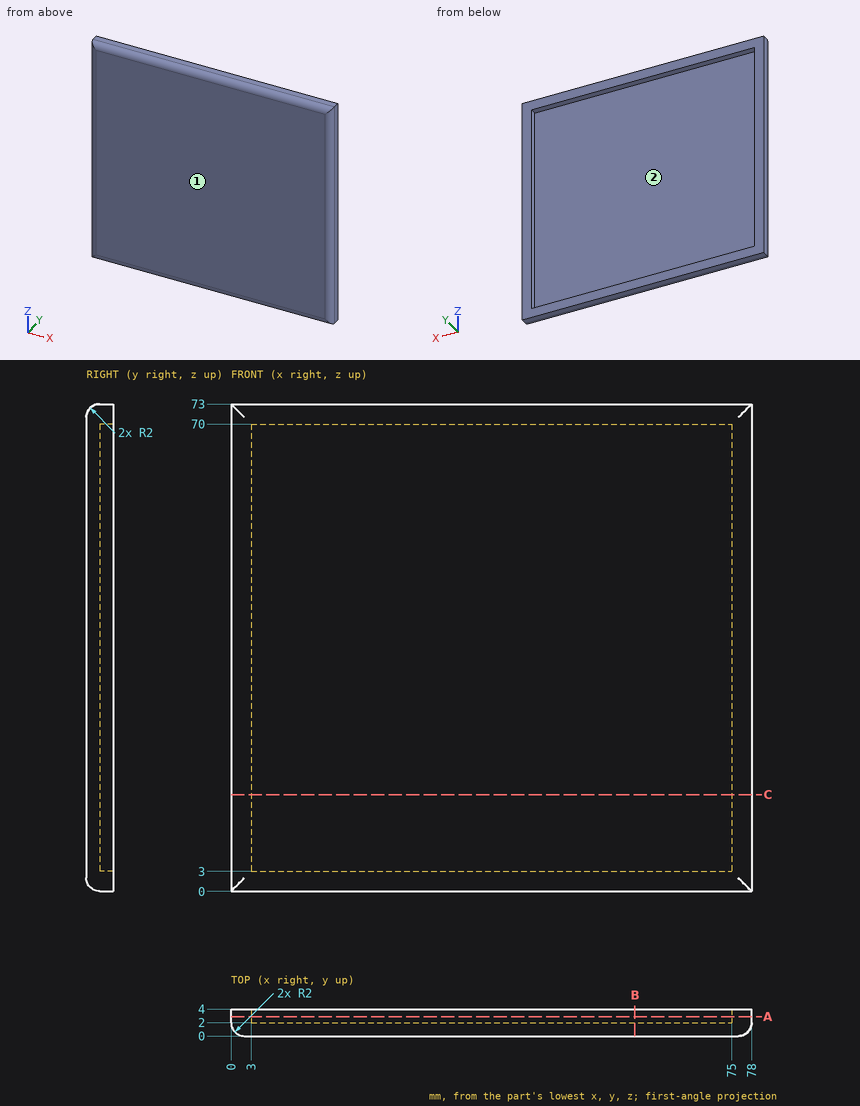
Study the drawing (mm; zero at the part's minimum x, y, z) and answer. Give positions to 0.01 mm unless a question says otherwise; leave off trailing zeros. Loops run counter-clockwise (first coordinate to the right, second up) from the corner with the lowest first, then second, coordinate; pieces in that order, holes last. Notation, with made-up numbers: M -23,3.5 L -8,3.5 A26 cw -8,39.5 Z; hole C 22,-31.75 d6. An arc over 180 degrees is marked long. Answer as CSV lines item,"result".
Item 1: Straight lines are drawn through the part: line 1 along Z through (x, y) = (23.5, 3.55); line 2 along X through (y, z) = (2.65, 45.5); line 3 along Y through (x, z) = (24.5, 5). For each, find the intervals that lie inside material, in ascending order. Write a range as [from, to].
Values follow:
line 1,"z = [0, 3], [70, 73]"
line 2,"x = [0, 3], [75, 78]"
line 3,"y = [0, 2]"
Item 2: The part is cut by section A-A (y = 2.9). Give the vertices of the cut face in (x, z).
Values follow:
outline,"M 0,0 L 78,0 L 78,73 L 0,73 Z; hole M 3,3 L 75,3 L 75,70 L 3,70 Z"
Item 3: The part is cut by section B-B (x = 60.5). Give the vertices of the cut face in (y, z), and give its area (3 significant figures).
Values follow:
outline,"M 0,2 A2 ccw 2,0 L 4,0 L 4,3 L 2,3 L 2,70 L 4,70 L 4,73 L 2,73 A2 ccw 0,71 Z"
area,"156 mm^2"
Item 4: The part is cut by section C-C (z = 14.5). Give the vertices of the cut face in (x, y), and give its area (3 significant figures).
Values follow:
outline,"M 0,2 A2 ccw 2,0 L 76,0 A2 ccw 78,2 L 78,4 L 75,4 L 75,2 L 3,2 L 3,4 L 0,4 Z"
area,"166 mm^2"
Item 5: Given pin 1 Ø12 at (x, z) = (23.5, 61) entering from +Y; pin 2 Ø1 at (x, y) = (22, 3) entering from -Z, each flat-ended and moving along its own axis, determine where each tip first touches the part or whether it passes through.
Values follow:
pin 1,"stops at y = 2"
pin 2,"stops at z = 0"
Item 6: The mould has two halves that part along Z. Classify the marked faces 1 and 2: released by +Z, released by -Z, zero draft, split by the parting line, or undercut.
Values follow:
face 1,"zero draft"
face 2,"undercut"
